```python
from build123d import *

# Parameters (mm, degrees)
F1_DEPTH = 20
F2_R     = 10
F3_DEPTH = 20


with BuildPart() as f1:
    # F0 (on Top) → F1 (new body)
    with BuildSketch(Plane.XY):
        with BuildLine():
            ThreePointArc((49.774727, -4.740946), (49.94365, -2.373147), (50, 0))
            ThreePointArc((50, 0), (49.94365, 2.373147), (49.774727, 4.740946))
            ThreePointArc((49.774727, 4.740946), (47.552826, 15.45085), (43.055258, 25.421345))
            ThreePointArc((43.055258, 25.421345), (40.45085, 29.389263), (37.481942, 33.092356))
            ThreePointArc((37.481942, 33.092356), (29.389263, 40.45085), (19.890144, 45.873546))
            ThreePointArc((19.890144, 45.873546), (15.45085, 47.552826), (10.872329, 48.803611))
            ThreePointArc((10.872329, 48.803611), (5.468978, 49.700003), (0, 50))
            ThreePointArc((0, 50), (-5.468978, 49.700003), (-10.872329, 48.803611))
            ThreePointArc((-10.872329, 48.803611), (-15.45085, 47.552826), (-19.890144, 45.873546))
            ThreePointArc((-19.890144, 45.873546), (-29.389263, 40.45085), (-37.481942, 33.092356))
            ThreePointArc((-37.481942, 33.092356), (-40.45085, 29.389263), (-43.055258, 25.421345))
            ThreePointArc((-43.055258, 25.421345), (-47.552826, 15.45085), (-49.774727, 4.740946))
            ThreePointArc((-49.774727, 4.740946), (-50, 0), (-49.774727, -4.740946))
            ThreePointArc((-49.774727, -4.740946), (-47.552826, -15.45085), (-43.055258, -25.421345))
            ThreePointArc((-43.055258, -25.421345), (-40.45085, -29.389263), (-37.481942, -33.092356))
            ThreePointArc((-37.481942, -33.092356), (-29.389263, -40.45085), (-19.890144, -45.873546))
            ThreePointArc((-19.890144, -45.873546), (-15.45085, -47.552826), (-10.872329, -48.803611))
            ThreePointArc((-10.872329, -48.803611), (0, -50), (10.872329, -48.803611))
            ThreePointArc((10.872329, -48.803611), (15.45085, -47.552826), (19.890144, -45.873546))
            ThreePointArc((19.890144, -45.873546), (29.389263, -40.45085), (37.481942, -33.092356))
            ThreePointArc((37.481942, -33.092356), (40.45085, -29.389263), (43.055258, -25.421345))
            ThreePointArc((43.055258, -25.421345), (47.552826, -15.45085), (49.774727, -4.740946))
        make_face()
        with BuildLine():
            ThreePointArc((43.055258, 25.421345), (47.552826, 15.45085), (49.774727, 4.740946))
            ThreePointArc((49.774727, 4.740946), (59.872276, 9.409519), (68.119041, 16.875907))
            Line((68.119041, 16.875907), (66.573956, 21.63119))
            Line((66.573956, 21.63119), (65.028871, 26.386472))
            ThreePointArc((65.028871, 26.386472), (53.968465, 27.57958), (43.055258, 25.421345))
        make_face()
        with BuildLine():
            ThreePointArc((68.119041, -16.875907), (59.872276, -9.409519), (49.774727, -4.740946))
            ThreePointArc((49.774727, -4.740946), (47.552826, -15.45085), (43.055258, -25.421345))
            ThreePointArc((43.055258, -25.421345), (53.968465, -27.57958), (65.028871, -26.386472))
            Line((65.028871, -26.386472), (66.573956, -21.63119))
            Line((66.573956, -21.63119), (68.119041, -16.875907))
        make_face()
        with BuildLine():
            ThreePointArc((19.890144, 45.873546), (29.389263, 40.45085), (37.481942, 33.092356))
            ThreePointArc((37.481942, 33.092356), (42.906913, 42.804502), (45.190053, 53.692263))
            Line((45.190053, 53.692263), (41.144968, 56.63119))
            Line((41.144968, 56.63119), (37.099883, 59.570116))
            ThreePointArc((37.099883, 59.570116), (27.450535, 54.034217), (19.890144, 45.873546))
        make_face()
        with BuildLine():
            ThreePointArc((45.190053, -53.692263), (42.906913, -42.804502), (37.481942, -33.092356))
            ThreePointArc((37.481942, -33.092356), (29.389263, -40.45085), (19.890144, -45.873546))
            ThreePointArc((19.890144, -45.873546), (27.450535, -54.034217), (37.099883, -59.570116))
            Line((37.099883, -59.570116), (41.144968, -56.63119))
            Line((41.144968, -56.63119), (45.190053, -53.692263))
        make_face()
        with BuildLine():
            ThreePointArc((0, 50), (5.468978, 49.700003), (10.872329, 48.803611))
            ThreePointArc((10.872329, 48.803611), (9.552567, 59.84962), (5, 70))
            Line((5, 70), (0, 70))
            Line((0, 70), (0, 50))
        make_face()
        with BuildLine():
            ThreePointArc((5, -70), (9.552567, -59.84962), (10.872329, -48.803611))
            ThreePointArc((10.872329, -48.803611), (0, -50), (-10.872329, -48.803611))
            ThreePointArc((-10.872329, -48.803611), (-9.552567, -59.84962), (-5, -70))
            Line((-5, -70), (0, -70))
            Line((0, -70), (5, -70))
        make_face()
        with BuildLine():
            ThreePointArc((-10.872329, 48.803611), (-5.468978, 49.700003), (0, 50))
            Line((0, 50), (0, 70))
            Line((0, 70), (-5, 70))
            ThreePointArc((-5, 70), (-9.552567, 59.84962), (-10.872329, 48.803611))
        make_face()
        with BuildLine():
            ThreePointArc((-37.099883, -59.570116), (-27.450535, -54.034217), (-19.890144, -45.873546))
            ThreePointArc((-19.890144, -45.873546), (-29.389263, -40.45085), (-37.481942, -33.092356))
            ThreePointArc((-37.481942, -33.092356), (-42.906913, -42.804502), (-45.190053, -53.692263))
            Line((-45.190053, -53.692263), (-41.144968, -56.63119))
            Line((-41.144968, -56.63119), (-37.099883, -59.570116))
        make_face()
        with BuildLine():
            ThreePointArc((-37.481942, 33.092356), (-29.389263, 40.45085), (-19.890144, 45.873546))
            ThreePointArc((-19.890144, 45.873546), (-27.450535, 54.034217), (-37.099883, 59.570116))
            Line((-37.099883, 59.570116), (-41.144968, 56.63119))
            Line((-41.144968, 56.63119), (-45.190053, 53.692263))
            ThreePointArc((-45.190053, 53.692263), (-42.906913, 42.804502), (-37.481942, 33.092356))
        make_face()
        with BuildLine():
            ThreePointArc((-65.028871, -26.386472), (-53.968465, -27.57958), (-43.055258, -25.421345))
            ThreePointArc((-43.055258, -25.421345), (-47.552826, -15.45085), (-49.774727, -4.740946))
            ThreePointArc((-49.774727, -4.740946), (-59.872276, -9.409519), (-68.119041, -16.875907))
            Line((-68.119041, -16.875907), (-66.573956, -21.63119))
            Line((-66.573956, -21.63119), (-65.028871, -26.386472))
        make_face()
        with BuildLine():
            ThreePointArc((-49.774727, 4.740946), (-47.552826, 15.45085), (-43.055258, 25.421345))
            ThreePointArc((-43.055258, 25.421345), (-53.968465, 27.57958), (-65.028871, 26.386472))
            Line((-65.028871, 26.386472), (-66.573956, 21.63119))
            Line((-66.573956, 21.63119), (-68.119041, 16.875907))
            ThreePointArc((-68.119041, 16.875907), (-59.872276, 9.409519), (-49.774727, 4.740946))
        make_face()
    extrude(amount=F1_DEPTH)

    # F2 (on face) → F3 (cut, through all)
    with BuildSketch(Plane.XY.offset(20)):
        Circle(F2_R)
    extrude(amount=-F3_DEPTH, mode=Mode.SUBTRACT)


solid = f1.part
```
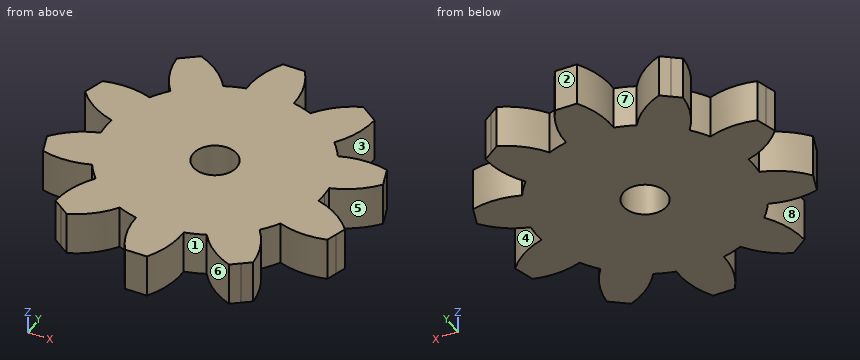
Input: part model. Units: mm. Frame: model coordinates. Face numbers are marked on the shaded views. A direction names the side the tool comes from. Give positions to 0.01 mm unless a question says otherwise; leave off trailing zeros. Loops run counter-clockwise (first coordinate to the right, second up) from the corner with the lowest first, then second, coordinate; pieces in that order, holes last. Notation, with made-up numbers: (28, -23.5) -> (49, -23.5) arc R22 cw to (49, 5.5) -> close; hole circle Ø6 at (-12.5, 13). An arc over 180 degrees is marked (long way). Use a Markdown table: item, result.
Q1. First-contact query: P1, Ø12, axis at y = -1, z = 5.5, coming from the -X side; P2, Ø12, axis at y = -4.5, z = 7.5, coming from the -X side; P3, Ø1, axis at y = -23, z = 10.5, coming from the +X side; P4, Ø6, axis at x = 6, y = 34.5, coming from the -Z side. Flat tips, straight axial feed; report the tip coordinate or a pass-through.
Entries:
| item | result |
|---|---|
| P1 | stops at x = -55.65 |
| P2 | stops at x = -61.43 |
| P3 | stops at x = 66.29 |
| P4 | stops at z = 0 |
Q2. Section query A-A, the plane x = 0. Return the cut outline in (y, z).
Entries:
| item | result |
|---|---|
| outline | (-70, 0) -> (-10, 0) -> (-10, 20) -> (-70, 20) -> close; (10, 0) -> (70, 0) -> (70, 20) -> (10, 20) -> close |
Q3. Pull-direction query (Y, two-part tool) for the marked faces 1, 2, 3 and 4; classes: pulls with the +Y half, pulls with the -Y half, needs draft (parallel to the pull), parting line crosses it, or undercut.
Entries:
| item | result |
|---|---|
| face 1 | pulls with the -Y half |
| face 2 | pulls with the +Y half |
| face 3 | undercut |
| face 4 | undercut |
Q4. Section query B-B, the plane x = 60. Return the cut outline in (y, z).
Entries:
| item | result |
|---|---|
| outline | (-27.35, 0) -> (-9.49, 0) -> (-9.49, 20) -> (-27.35, 20) -> close; (9.49, 0) -> (27.35, 0) -> (27.35, 20) -> (9.49, 20) -> close |
Q5. Access query for the marked faces 5, 6, 7 and 8. Directions: +Z, -Z, +X, -X, +Y, -Y. A direction counts if a zero-diameter tool reaches every point of the face in a straight line with its end or side. Return the directions, or none.
Entries:
| item | result |
|---|---|
| face 5 | +Z, -Z, +X |
| face 6 | +Z, -Z, -Y |
| face 7 | +Z, -Z, +Y |
| face 8 | +Z, -Z, -X |
Q6. Section query D-D, the plane x = 29. Return the cut outline in (y, z), plus the area to 3 significant figures.
Entries:
| item | result |
|---|---|
| outline | (-55.2, 0) -> (55.2, 0) -> (55.2, 20) -> (-55.2, 20) -> close |
| area | 2,210 mm² |
Q7. Section query C-C, the plane y = -36. Return the cut outline in (x, z), plus the area to 3 significant figures.
Entries:
| item | result |
|---|---|
| outline | (-39.53, 0) -> (39.53, 0) -> (39.53, 20) -> (-39.53, 20) -> close |
| area | 1,580 mm² |
Q8. Ray query, probe 1 along Y at (x, z) = (0, 12.5); probe 2 along X at (y, z) = (-51.5, 9.5); probe 3 along Y at (x, z) = (-54, 2). Return the intervals inside material, ascending. Write a range as from..to.
Entries:
| item | result |
|---|---|
| probe 1 | y = -70..-10, 10..70 |
| probe 2 | x = -45..-24.58, -10.86..10.86, 24.58..45 |
| probe 3 | y = -27.58..-6.25, 6.25..27.58 |
